from build123d import *

# Parameters (mm, degrees)
BOSS_EXTRUDE1_DEPTH = 150
SKETCH2_R           = 2.5
CUT_EXTRUDE1_DEPTH  = 154.493688795


with BuildPart() as part:
    # Sketch1 → Boss-Extrude1 (new body)
    with BuildSketch(Plane(origin=(0, 0, 0), x_dir=(0, 0, -1), z_dir=(1, 0, 0))):
        Polygon((-14.25, 0), (15.75, 0), (15.75, 1.5), (1.5, 1.5), (1.5, 30), (0, 30), (0, 1.5), (-14.25, 1.5), align=None)
    extrude(amount=BOSS_EXTRUDE1_DEPTH)

    # Sketch2 → Cut-Extrude1 (cut, through all)
    with BuildSketch(Plane(origin=(0, 1.5, 0), x_dir=(1, 0, 0), z_dir=(0, 1, 0))):
        with Locations(Location((12.75, -6.75, 0), (0, 0, 270))):
            Circle(SKETCH2_R)
        with Locations(Location((12.75, 8.25, 0), (0, 0, 270))):
            Circle(SKETCH2_R)
        with Locations(Location((53.55, 8.25, 0), (0, 0, 270))):
            Circle(SKETCH2_R)
        with Locations(Location((53.55, -6.75, 0), (0, 0, 270))):
            Circle(SKETCH2_R)
        with Locations(Location((96.45, -6.75, 0), (0, 0, 90))):
            Circle(SKETCH2_R)
        with Locations(Location((96.45, 8.25, 0), (0, 0, 90))):
            Circle(SKETCH2_R)
        with Locations(Location((137.25, 8.25, 0), (0, 0, 90))):
            Circle(SKETCH2_R)
        with Locations(Location((137.25, -6.75, 0), (0, 0, 90))):
            Circle(SKETCH2_R)
    extrude(amount=-CUT_EXTRUDE1_DEPTH, mode=Mode.SUBTRACT)


solid = part.part
Work out the finished part from the listing and answer in its coordinate system (mm). A direction names the side the tool comes from. Give positions to 0.01 mm unless a question says otherwise; leave off trailing zeros. Loops run counter-clockwise (first coordinate to the right, second up) from the corner with the lowest first, then second, coordinate; pieces in that order, holes last. Notation, with made-up numbers: M 59.25,63 L 113.25,63 A15 cw 113.25,85 Z; hole C 28.5,17 d5. An arc over 180 degrees is marked long. Use CSV: the item, a comma, the result in double quotes.
1) Find section C-C on y = 12.25. Write down the section's boundary in (x, z), plus the area to 3 significant figures.
Answer:
outline,"M 0,-1.5 L 150,-1.5 L 150,0 L 0,0 Z"
area,"225 mm^2"
2) Find section A-A on x = 96.45. Write down the section's boundary in (y, z), plus the area to 4 significant figures.
Answer:
outline,"M 0,-15.75 L 1.5,-15.75 L 1.5,-10.75 L 0,-10.75 Z; M 0,-5.75 L 1.5,-5.75 L 1.5,-1.5 L 30,-1.5 L 30,0 L 1.5,0 L 1.5,4.25 L 0,4.25 Z; M 0,9.25 L 1.5,9.25 L 1.5,14.25 L 0,14.25 Z"
area,"72.75 mm^2"
3) Find section B-B on z = 6.75. Write down the section's boundary in (x, y).
Answer:
outline,"M 0,0 L 10.25,0 L 10.25,1.5 L 0,1.5 Z; M 15.25,0 L 51.05,0 L 51.05,1.5 L 15.25,1.5 Z; M 56.05,0 L 93.95,0 L 93.95,1.5 L 56.05,1.5 Z; M 98.95,0 L 134.75,0 L 134.75,1.5 L 98.95,1.5 Z; M 139.75,0 L 150,0 L 150,1.5 L 139.75,1.5 Z"
4) Given P1, Ø11.5, axis at x = 51.5, z = 6, coming from the +Y side; P2, Ø8.5, axis at x = 67, y = 15, coming from the +Z side; P3, Ø2, axis at x = 67.5, y = 27, coming from the -Z side, each flat-ended and moving along its own axis, determine where each tip first touches the part or whether it passes through.
Answer:
P1,"y = 1.5"
P2,"z = 0"
P3,"z = -1.5"
5) Which of the six approach directions +Z, -Z, +X, -X, +Y, -Y give full straight-line access (tool end or side, diameter ignored) to faces 1 (the cylindrical face through (10.31, 0.76, -8.79)), 2 (the flat face through (74, 1.5, -9)), 3 (the flat face through (74, 16, 0))?
Answer:
face 1,"+Y, -Y"
face 2,"-Z, +X, -X, +Y"
face 3,"+Z, +X, -X, +Y"
6) Consider L1, parallel to Z at x = 96.45, y = 0.55; L2, parallel to X at y = 0.4, z = -8.25; L3, parallel to Y at x = 112, z = 1.5. Determine where each line is inside the solid, lowest interval first.
Answer:
L1,"-15.75 to -10.75, -5.75 to 4.25, 9.25 to 14.25"
L2,"0 to 10.25, 15.25 to 51.05, 56.05 to 93.95, 98.95 to 134.75, 139.75 to 150"
L3,"0 to 1.5"
